```python
from build123d import *

# Parameters (mm, degrees)
SKETCH2_R           = 9.52900057
CUT_EXTRUDE2_DEPTH  = 62
SKETCH3_R           = 12
SKETCH3_R_2         = 6
BOSS_EXTRUDE1_DEPTH = 2.5


with BuildPart() as part:
    # Sketch1 → Revolve1 (revolve)
    with BuildSketch(Plane.XY):
        Polygon((0, 0), (0, 37.5), (1, 37.5), (2, 34.752522581), (4, 34.752522581), (5, 37.5), (6, 37.5), (6, 0), align=None)
    revolve(axis=Axis((0, 0, 0), (1, 0, 0)))

    # Sketch2 → Cut-Extrude2 (cut)
    with BuildSketch(Plane(origin=(6, 0, 0), x_dir=(0, 0, -1), z_dir=(1, 0, 0))):
        Circle(SKETCH2_R)
    extrude(amount=-CUT_EXTRUDE2_DEPTH, mode=Mode.SUBTRACT)

    # Sketch3 → Boss-Extrude1 (add)
    with BuildSketch(Plane(origin=(6, 0, 0), x_dir=(0, 0, -1), z_dir=(1, 0, 0))):
        Circle(SKETCH3_R)
        Circle(SKETCH3_R_2, mode=Mode.SUBTRACT)
    extrude(amount=BOSS_EXTRUDE1_DEPTH)

    # Mirror1: part across plane


with BuildPart() as part_1:
    add(part.part)
    add(part.part.mirror(Plane(origin=(0, 0, 0), x_dir=(0, 0, 1), z_dir=(1, 0, 0))))


solid = part_1.part
```
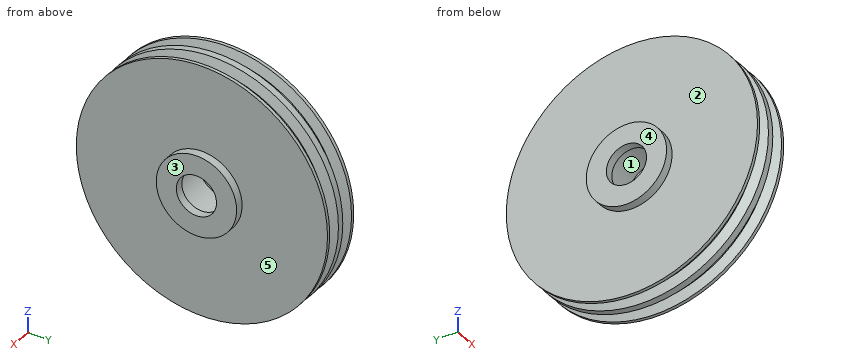
Read the model definition and answer for the solid it produces. Units are mm, in the model's axes. Face numbers are marked on the shaded views. A direction names the side the tool comes from. Coordinates: 2 decimals unless noted, no trailing zeros. Return JSON: item names as keys, results as strings.
1. Find the intervals of material crossed by line 1 along Y through (x, z) = (6.85, 0); line 2 along X through (y, z) = (12, -2.5); line 3 along Y through (x, z) = (2.75, 14.5), in increasing order. Write a range as from..to.
Found:
{"line 1": "-12..-6, 6..12", "line 2": "-6..6", "line 3": "-31.58..31.58"}
2. Determine the mould class of the marked faces 1, 2 and 3 for opening direction X: pulls with the +X half, pulls with the -X half, needs draft (parallel to the pull), parting line crosses it, or undercut.
Found:
{"face 1": "undercut", "face 2": "pulls with the -X half", "face 3": "pulls with the +X half"}
3. Each of these flat-tipped pins is pushed along its axis until it touches: P1, Ø2, axis at y = 14, z = -22, coming from the -X side; P2, Ø15.5, axis at y = 0, z = 0, coming from the -X side; P3, Ø4, axis at x = -5, z = 11.5, coming from the +Y side; P4, Ø4, axis at y = 12, z = -25, coming from the +X side. Where does it stop, or does it pass through?
Found:
{"P1": "x = -6", "P2": "x = -8.5", "P3": "y = 36.28", "P4": "x = 6"}
4. A tool of negligible diameter and unlimited length cuts with its end or side. For the marked faces 4 and 5, from which of +Z, -Z, +X, -X, +Y, -Y can it reach the whole face along a straight path? Write none if from no direction.
Found:
{"face 4": "+Z, -Z, -X, +Y, -Y", "face 5": "+X"}
